```python
from build123d import *

# Parameters (mm, degrees)
F1_DEPTH = 292
F3_DEPTH = 80
F4_R     = 5
F5_DEPTH = 25
F6_R     = 5
F7_DEPTH = 25


with BuildPart() as f1:
    # F0 (on Front) → F1 (new body)
    with BuildSketch(Plane.XZ):
        with BuildLine():
            Line((-10.877076, 89.111448), (-90.877076, 89.111448))
            Line((-90.877076, 89.111448), (-90.877076, 9.111448))
            ThreePointArc((-90.877076, 9.111448), (-83.806008, 12.04038), (-80.877076, 19.111448))
            Line((-80.877076, 19.111448), (-80.877076, 69.111448))
            ThreePointArc((-80.877076, 69.111448), (-77.948143, 76.182516), (-70.877076, 79.111448))
            Line((-70.877076, 79.111448), (-20.877076, 79.111448))
            ThreePointArc((-20.877076, 79.111448), (-13.806008, 82.04038), (-10.877076, 89.111448))
        make_face()
    extrude(amount=F1_DEPTH)

    # F2 (on face) → F3 (cut)
    with BuildSketch(Plane(origin=(-90.877076, 0, 0), x_dir=(0, -1, 0), z_dir=(-1, 0, 0))):
        Polygon((292, 9.111448), (292, 89.111448), (201.576449, 9.111448), align=None)
        Polygon((0, 9.111448), (90.423551, 89.111448), (0, 89.111448), align=None)
    extrude(amount=-F3_DEPTH, mode=Mode.SUBTRACT)

    # F4 (on face) → F5 (cut)
    with BuildSketch(Plane(origin=(-90.877076, 0, 0), x_dir=(0, -1, 0), z_dir=(-1, 0, 0))):
        with Locations((212, 49.111448)):
            Circle(F4_R)
        with Locations((80, 49.111448)):
            Circle(F4_R)
    extrude(amount=-F5_DEPTH, mode=Mode.SUBTRACT)

    # F6 (on face) → F7 (cut)
    with BuildSketch(Plane.XY.offset(89.111448)):
        with Locations((-60.877076, -242)):
            Circle(F6_R)
        with Locations((-60.877076, -130.423551)):
            Circle(F6_R)
        with Locations((-30.877076, -130.423551)):
            Circle(F6_R)
        with Locations((-30.877076, -242)):
            Circle(F6_R)
    extrude(amount=-F7_DEPTH, mode=Mode.SUBTRACT)


solid = f1.part
```
The listing builds one solid part. Answer for the finished solid, in the listing's coordinates (mm). A direction names the side the tool comes from. Give positions to 0.01 mm unless a question says otherwise; leave off trailing zeros. Write each loop counter-clockwise with the first axis right and the second up, starting at its lowest first coordinate (ties: lowest second). Pieces come first, ordered by that corner, then holes. Notation, with made-up numbers: (-4, 69.25) - (52, 69.25) arc R16 cw to (52, 81.25) - close; hole circle Ø5 at (73, 87). An arc over 180 degrees is marked (long way). Use one line per item in the form item = value. Start each with the question number.
1) Find section A-A on y = -167.5. Determine the outline of the cut face in (x, z), plus the area to 3 significant figures.
2) Find section D-D on y = -35.5. Determine the outline of the cut face in (x, z).
3) Consider line 1 along Y through (x, z) = (-32.5, 84.5); line 2 along Z through (x, y) = (-26, -98.5); line 3 along X through (y, z) = (-98.5, 39). Determine where each line is inside the solid, lowest interval first. Write a range as from..to.
4) A tool of negligible diameter and unlimited length cuts with its end or side. For faces 4 (the face through (-80.877, -139, 44)), 5 (the face through (-28.57, -134.86, 84.18)), from which of +Z, -Z, +X, -X, +Y, -Y can it reach the whole face along a straight path? Write none if from no direction.
5) Find section C-C on z = 33. Determine the outline of the cut face in (x, y).
6) Find section B-B on y = -242. Determine the outline of the cut face in (x, z).
7) Flat-ended cylindrical pins translate along their axes: pin 1 Ø2 at (y, z) = (-170, 58) entering from +X; pin 2 Ø12 at (x, y) = (-44, -237) entering from -Z. Find the tip coordinate at first contact, or state that the pin passes through.
8) The mould has two halves that part along X. Classify faces 1 (the face through (-85.95, -216.62, 47.2)), 2 (the face through (-90.877, -144, 50)), 3 (the face through (-31.528, -237.043, 84.181)): pulls with the +X half, pulls with the -X half, needs draft (parallel to the pull), parting line crosses it, or undercut.
Geometry results:
q1.outline = (-90.88, 9.11) arc R10 ccw to (-80.88, 19.11) - (-80.88, 69.11) arc R10 cw to (-70.88, 79.11) - (-20.88, 79.11) arc R10 ccw to (-10.88, 89.11) - (-90.88, 89.11) - close
q1.area = 1,480 mm2
q2.outline = (-90.88, 9.11) arc R10 ccw to (-80.88, 19.11) - (-80.88, 40.52) - (-90.88, 40.52) - close
q3.line_1 = -286.79..-246.73, -237.27..-135.15, -125.69..-85.21
q3.line_2 = 79.11..89.11
q3.line_3 = -90.88..-80.88
q4.face_4 = -Z, +X, +Y, -Y
q4.face_5 = +Z, -Z
q5.outline = (-90.88, -228.58) - (-80.88, -228.58) - (-80.88, -27) - (-90.88, -27) - close
q6.outline = (-90.88, 44.88) - (-80.88, 44.88) - (-80.88, 69.11) arc R10 cw to (-70.88, 79.11) - (-65.88, 79.11) - (-65.88, 89.11) - (-90.88, 89.11) - close; (-55.88, 79.11) - (-35.88, 79.11) - (-35.88, 89.11) - (-55.88, 89.11) - close; (-25.88, 79.11) - (-20.88, 79.11) arc R10 ccw to (-10.88, 89.11) - (-25.88, 89.11) - close
q7.pin_1 = -80.88
q7.pin_2 = 79.11
q8.face_1 = needs draft
q8.face_2 = pulls with the -X half
q8.face_3 = undercut
